```python
from build123d import *

# Parameters (mm, degrees)
F3_D = 18


with BuildPart() as f1:
    # F0 (on Front) → F1 (revolve)
    with BuildSketch(Plane.XZ):
        Polygon((10.919107, 50), (0, 20), (0, 0), (24, 0), (24, 12), (15, 12), (15, 50), align=None)
    revolve(axis=Axis((12, 0, 0), (-1, 0, 0)))

    # F3 (through all)
    with Locations(Plane(origin=(0, 0, 0), x_dir=(0, 1, 0), z_dir=(-1, 0, 0))):
        with Locations((0, 0)):
            Hole(F3_D / 2)


solid = f1.part
```
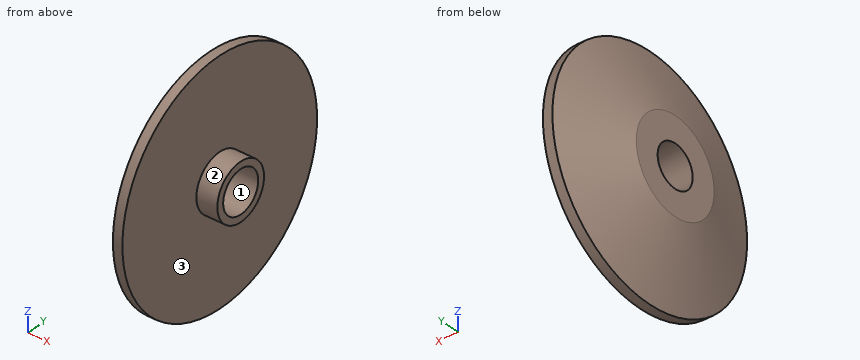
Here's how the part is built. I have some questions about the finished solid (model axes, mm). Face numbers are marked on the shaded views. Round coordinates to 2 decimals unless told otherwise and drop trailing zeros. Order: outer loops, then holes, each group sorted by start corner. A loop starts at its lowest first (then second) coordinate and runs counter-clockwise, first axis right, second up. Notation, with made-up numbers: (-36, 6.5) -> (20, 6.5) arc R12 ccw to (20, 25.5) -> close; hole circle Ø4 at (68, 7). An arc over 180 degrees is marked (long way). Use a Markdown table: item, result. Add a question column.
(1) For pin 1 Ø12 at (x, z) = (11.5, 36) entering from +Y; pin 2 Ø8 at (x, z) = (11, -5.5) entering from -Y; pin 3 Ø10 at (x, y) = (19, 26.5) entering from -Z; pin 4 Ø12 at (x, y) = (5.5, 1) entering from +Z, each with a flat end and sliding along its axis, tell me the tip position at first contact or that it passes through.
(2) I need wall thicknesses on line 1 along Y through (x, z) = (11, 0.5); line 2 along Z through (x, y) = (11.75, -6.5); line 3 along Z through (x, y) = (11, -2.5). Which ranges of each line are inside material? Lowest first, please.
(3) Suppose I cut it at C-C, the plane x = 20.5. Please give me the cut outline in (y, z), and give its area (3 significant figures).
(4) Suppose I cut it at D-D, the plane x = 5.75. Please give me the cut outline in (y, z).
(5) Suppose I cut it at A-A, the plane y = 0. Please give me the cut outline in (x, z).
(6) If we mould it in two halves opening along Y, with no side actions, what happens to the marked faces 1, 2 and 3? For each: released by +Y, released by -Y, zero draft, split by the parting line, or undercut.
Verdict:
| question | item | result |
|---|---|---|
| 1 | pin 1 | y = 40 |
| 1 | pin 2 | y = -49.98 |
| 1 | pin 3 | z = -44.13 |
| 1 | pin 4 | z = 50 |
| 2 | line 1 | -50 to -8.99, 8.99 to 50 |
| 2 | line 2 | -49.58 to -6.22, 6.22 to 49.58 |
| 2 | line 3 | -49.94 to -8.65, 8.65 to 49.94 |
| 3 | outline | circle Ø24 at (0, 0); hole circle Ø18 at (0, 0) |
| 3 | area | 198 mm2 |
| 4 | outline | circle Ø71.6 at (0, 0); hole circle Ø18 at (0, 0) |
| 5 | outline | (0, -20) -> (10.92, -50) -> (15, -50) -> (15, -12) -> (24, -12) -> (24, -9) -> (0, -9) -> close; (0, 9) -> (24, 9) -> (24, 12) -> (15, 12) -> (15, 50) -> (10.92, 50) -> (0, 20) -> close |
| 6 | face 1 | undercut |
| 6 | face 2 | split by the parting line |
| 6 | face 3 | zero draft |
